Part model, mm, in its own coordinate system. Face numbers are marked on the shaded views. A direction names the side the tool comes from. Coordinates: 2 decimals unless noted, no trailing zeros. Loops run counter-clockwise (first coordinate to the right, second up) from the corner with the lowest first, then second, coordinate; pieces in that order, holes last. Notation, with made-up numbers: (40, 37.25) - (90, 37.25) arc R13 ccw to (90, 54.25) - close; hole circle Ø7 at (-4.5, -34.5). An arc over 180 degrees is marked (long way). Use a Markdown table: item, result. Add a question column.
1. Band-saw the part on B-B, the plane x = 32. Give the cut face in (y, z).
2. Band-saw the part on D-D, the plane x = -22.5. Give the cut face in (y, z).
3. Band-saw the part on A-A, the plane x = 42. Give the cut face in (y, z).
4. Band-saw the part on C-C, the plane x = -10.5. Give the cut face in (y, z).
5. Drop flat-ended pins along their axis: pin 1 (4 mm diameter, centred on x = 1.5, z = -3, fed in from +Y); pin 2 (1.5 mm diameter, centred on x = 25.5, y = 9, fed in from -Z); pin 3 (8 mm diameter, centred on x = -12.5, z = 11, fed in from -Y). Give the stop position or say it passes through.
6. 3-axis set-ups, long thin cutter, end or side, ignore diameter. For the marked faces 4, 5 and 6: which of +Z, -Z, +X, -X, +Y, -Y reach the whole face in a straight line?
7. Pull direction X, two halves, no side cores. Call the marked faces 1, 2 and 3: pulls with the +X half, pulls with the -X half, needs draft (parallel to the pull), parting line crosses it, or undercut.
8. Wall check: probe 1 along X at (y, z) = (4.25, 0); probe 2 along X at (y, z) = (8, -1.5); probe 3 along X at (y, z) = (0, -3.5). Give the ranges that are in metal, low to high. Write a range as [from, to].
Autodesk Inventor part; units mm, degrees
ref_plane "YZ Plane" through (0, 0, 0) normal (1, 0, 0) x (0, 1, 0)
ref_plane "XY Plane" through (0, 0, 0) normal (0, 0, 1) x (1, 0, 0)
sketch "Эскиз2" plane through (0, 0, 0) normal (0, 0, 1) x (1, 0, 0)
  line L0 (-45, 0) -> (-45, 9)
  line L1 (-27.75, 9) -> (-45, 9)
  line L2 (-26, 7.25) -> (-20, 7.25)
  line L3 (-20, 7.25) -> (-20, 14)
  line L4 (-19, 15) -> (20, 15)
  line L5 (-26, 7.25) -> (-27.75, 9)
  line L6 (50, 10) -> (50, 0)
  line L7 (50, 10) -> (20, 10)
  line L8 (20, 10) -> (20, 14)
  line L9 (-45, 0) -> (50, 0)
  line L10 (-20, 14) -> (-20, 15)
  line L11 (-20, 15) -> (-19, 15)
  line L12 (20, 15) -> (20, 14)
  point P0 (0, 0)
  point P1 (0, 15)
  dimension "d1" = 9
  dimension "d15" = 6
  dimension "d16" = 19
  dimension "d22" = 10
  dimension "d23" = 20
  dimension "d41" = 25
  dimension "d42" = 17.25
  dimension "d57" = 20
  dimension "d58" = 70
revolve "Вращение1" add sketch "Эскиз2" angle 360 about axis through (-45, 0, 0) along (1, 0, 0)
sketch "Эскиз3" plane through (0, 0, 0) normal (0, 1, 0) x (-1, 0, 0)
  line L0 (-50, -10) -> (-30, -10)
  line L1 (-30, -10) -> (-30, -6.5)
  line L2 (-30, -6.5) -> (-50, -6.5)
  line L3 (-50, -6.5) -> (-50, -10)
  line L4 (-50, 10) -> (-30, 10)
  line L5 (-30, 10) -> (-30, 6.5)
  line L6 (-30, 6.5) -> (-50, 6.5)
  line L7 (-50, 6.5) -> (-50, 10)
  point P0 (0, 0)
extrude "Выдавливание1" cut sketch "Эскиз3" along normal mid plane 44.25
sketch "Эскиз4" plane through (0, 0, 0) normal (0, 0, 1) x (1, 0, 0)
  line L0 (50, 7.5993) -> (50, -7.5993)
  point P0 (0, 0)
  point P1 (42, 0)
hole "Отверстие1" at (42, 0, 0) direction (0, 0, -1) diameter 4 end through all both
thread "Резьба1"
chamfer "Фаска1" distance 2.5 angle 45 1 edges at (-45, -9, 0)
ref_plane "РабПлоскость1" through (0, 15, 0) normal (0, 1, 0) x (-1, 0, 0)
fillet "Сопряжение1" radius 1.6 1 edges at (-20, -7.25, 0)
fillet "Сопряжение2" radius 1 1 edges at (-26, -7.25, 0)
chamfer "Фаска2" distance 1 angle 45 2 edges at (20, -15, 0) (-20, -15, 0)
sketch "Эскиз6" plane through (0, 15, 0) normal (0, 1, 0) x (-1, 0, 0)
  point P0 (0, 0)
  point P1 (0, 0)
hole "Отверстие3" at (0, 15, 0) direction (0, -1, 0) diameter 10 depth 15 tip angle 118
properties part number "вал"
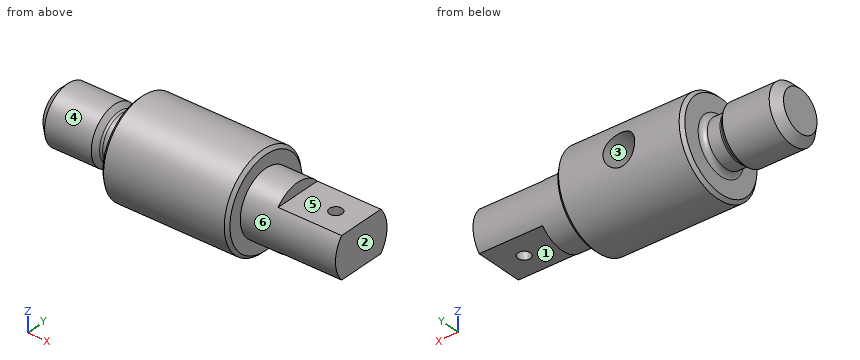
Geometry check:
| question | item | result |
|---|---|---|
| 1 | outline | (-7.6, -6.5) - (7.6, -6.5) arc R10 ccw to (7.6, 6.5) - (-7.6, 6.5) arc R10 ccw to start |
| 2 | outline | circle Ø14.5 at (0, 0) |
| 3 | outline | (-7.6, -6.5) - (-2, -6.5) - (-2, 6.5) - (-7.6, 6.5) arc R10 ccw to start; (2, -6.5) - (7.6, -6.5) arc R10 ccw to (7.6, 6.5) - (2, 6.5) - close |
| 4 | outline | circle Ø30 at (0, 0) |
| 5 | pin 1 | stops at y = 14.54 |
| 5 | pin 2 | stops at z = -5.65 |
| 5 | pin 3 | stops at y = -13.27 |
| 6 | face 4 | -X |
| 6 | face 5 | +Z, +X, +Y, -Y |
| 6 | face 6 | +X |
| 7 | face 1 | needs draft |
| 7 | face 2 | pulls with the +X half |
| 7 | face 3 | undercut |
| 8 | probe 1 | x = [-45, -5], [5, 50] |
| 8 | probe 2 | x = [-43.36, -26.89], [-20.17, -4.77], [4.77, 50] |
| 8 | probe 3 | x = [-45, -3.57], [3.57, 40], [44, 50] |
